Verification items for the finished model (mm, model axes). A direction names the side the tool comes from. Round coordinates to 2 decimals unless told otherwise and drop trailing zeros. Order: outer loops, then holes, each group sorted by start corner. A loop starts at its lowest first (then second) coordinate and runs counter-clockwise, first axis right, second up. Notation, with made-up numbers: (75.25, 87) -> (82.25, 87) arc R13 cw to (82.25, 96) -> close; hole circle Ø7 at (10, 29.5). An arc over 180 degrees is marked (long way). Put each result on its own line as item: value.
from build123d import *

# Parameters (mm, degrees)
BOSS_EXTRUDE1_DEPTH = 15
CHAMFER1_SIZE       = 2.5
SKETCH2_R           = 1.4
CUT_EXTRUDE1_DEPTH  = 15
CHAMFER2_SIZE       = 2
SKETCH3_R           = 1.4
CUT_EXTRUDE2_DEPTH  = 47.129659115
CUT_EXTRUDE3_DEPTH  = 25


with BuildPart() as part:
    # Sketch1 → Boss-Extrude1 (new body)
    with BuildSketch(Plane.XY):
        with BuildLine():
            Line((-19, 0), (-19, -4))
            Line((-19, -4), (-34, -4))
            Line((-34, -4), (-34, 0))
            Line((-34, 0), (-22.883234523, 0))
            ThreePointArc((-22.883234523, 0), (-17.861391251, 14.304304416), (-5, 22.33030278))
            Line((-5, 22.33030278), (-5, 27.33030278))
            Line((-5, 27.33030278), (-1, 27.33030278))
            Line((-1, 27.33030278), (-1, 18.33030278))
            Line((-1, 18.33030278), (-5, 18.33030278))
            ThreePointArc((-5, 18.33030278), (-15.099668871, 11.532562595), (-19, 0))
        make_face()
    extrude(amount=BOSS_EXTRUDE1_DEPTH)

    # Chamfer1
    chamfer1_edges = [part.edges().sort_by_distance(p)[0] for p in [
        (-34, -2, 0),
        (-34, -2, 15),
    ]]
    chamfer(chamfer1_edges, length=CHAMFER1_SIZE)

    # Sketch2 → Cut-Extrude1 (cut)
    with BuildSketch(Plane.ZY.offset(5)):
        with Locations(Location((2.8, 24.83030278, 0), (0, 0, 270))):
            Circle(SKETCH2_R)
        with Locations(Location((12.2, 24.83030278, 0), (0, 0, 270))):
            Circle(SKETCH2_R)
    extrude(amount=-CUT_EXTRUDE1_DEPTH, mode=Mode.SUBTRACT)

    # Chamfer2
    chamfer2_edges = [part.edges().sort_by_distance(p)[0] for p in [
        (-3, 27.33030278, 0),
        (-3, 27.33030278, 15),
    ]]
    chamfer(chamfer2_edges, length=CHAMFER2_SIZE)

    # Sketch3 → Cut-Extrude2 (cut, through all)
    with BuildSketch(Plane(origin=(0, 0, 0), x_dir=(1, 0, 0), z_dir=(0, 1, 0))):
        with Locations(Location((-28.441617262, -7.5, 0), (0, 0, 270))):
            Circle(SKETCH3_R)
    extrude(amount=-CUT_EXTRUDE2_DEPTH, mode=Mode.SUBTRACT)

    # Sketch4 → Cut-Extrude3 (cut)
    with BuildSketch(Plane.XZ.offset(4)):
        Polygon((-24.636069701, 0), (-34, 6.600391812), (-34, 2.5), (-31.5, 0), align=None)
    extrude(amount=-CUT_EXTRUDE3_DEPTH, mode=Mode.SUBTRACT)


solid = part.part
Item 1: Section check A-A on z = 7.5. Record the boundary of the cut face in (x, y), then the cut area to 3 significant figures.
Check sheet entries:
outline: (-34, -4) -> (-29.84, -4) -> (-29.84, 0) -> (-34, 0) -> close; (-27.04, -4) -> (-19, -4) -> (-19, 0) arc R19 cw to (-5, 18.33) -> (-1, 18.33) -> (-1, 27.33) -> (-5, 27.33) -> (-5, 22.33) arc R22.88 ccw to (-22.88, 0) -> (-27.04, 0) -> close
area: 193 mm^2
Item 2: Release check for a two-part mould opening along X. For faces 4 (the cylindrical face through (-29.81, -1.97, 7.2)), 5 (the cylindrical face through (-18, 14.13, 7.4)), 6 (the flat face through (-1, 23, 7)), 7 (the flat face through (-3, 18.33, 7)) record: +X half, -X half, draft (parallel to the pull), parting line (faces both ways), or undercut.
Check sheet entries:
face 4: undercut
face 5: -X half
face 6: +X half
face 7: draft
Item 3: Section check C-C on y = 14. Record the boundary of the cut face in (x, z), then the cut area to 3 significant figures.
Check sheet entries:
outline: (-18.1, 0) -> (-12.85, 0) -> (-12.85, 15) -> (-18.1, 15) -> close
area: 78.8 mm^2
Item 4: Section check B-B on z = 14.25. Record the boundary of the cut face in (x, y).
Check sheet entries:
outline: (-32.25, -4) -> (-19, -4) -> (-19, 0) arc R19 cw to (-5, 18.33) -> (-1, 18.33) -> (-1, 26.08) -> (-5, 26.08) -> (-5, 22.33) arc R22.88 ccw to (-22.88, 0) -> (-32.25, 0) -> close
Item 5: Section check D-D on x = -22. Record the boundary of the cut face in (y, z).
Check sheet entries:
outline: (-4, 0) -> (6.3, 0) -> (6.3, 15) -> (-4, 15) -> close
Item 6: Material ranges on L1, parallel to X at y = -1.95, z = 7.5; L2, parallel to Y at x = -24, z = 7; L3, parallel to X at y = 19.5, z = 13.5, recorded low to high. Write a range as [from, to].
Check sheet entries:
L1: x = [-34, -29.84], [-27.04, -19]
L2: y = [-4, 0]
L3: x = [-11.97, -1]
Item 7: Tool access check on faces 1 (the flat face through (-19, -2, 7)), 2 (the flat face through (-29.25, -2.03, 3.25)), 3 (the flat face through (-5, 25, 7)). Record the directions out of +Z, -Z, +X, -X, +Y, -Y that give a thin tool (end or side, any length) a straight path to the whole face; none if there is none.
Check sheet entries:
face 1: +Z, -Z, +X, -Y
face 2: -Z, -X, +Y, -Y
face 3: +Z, -Z, -X, +Y
Item 8: Gauge pin test, flat ends, axial feed: pin 1 Ø8 at (y, z) = (6.5, 13) entering from -X; pin 2 Ø1.5 at (y, z) = (24.5, 7.5) entering from -X; pin 3 Ø3 at (y, z) = (6.5, 9.5) entering from -X. Record the tip position at first contact, or that the pin passes through.
Check sheet entries:
pin 1: stops at x = -22.75
pin 2: stops at x = -5
pin 3: stops at x = -22.33
